Model file for the job. Use its own axes, mm. Face numbers are marked on the shaded views. A direction names the side the tool comes from. Give positions to 0.01 mm unless a question says otherwise; leave off trailing zeros. Write each loop counter-clockwise with the first axis right and the second up, starting at its lowest first coordinate (ties: lowest second). Pieces come first, ordered by that corner, then holes. Notation, with made-up numbers: (7, -17) - (13, -17) arc R21 ccw to (13, -9) - close; hole circle Ø1 at (4.5, -0.75). An arc over 180 degrees is marked (long way). Use CSV: the item, a comma, the result in double quotes.
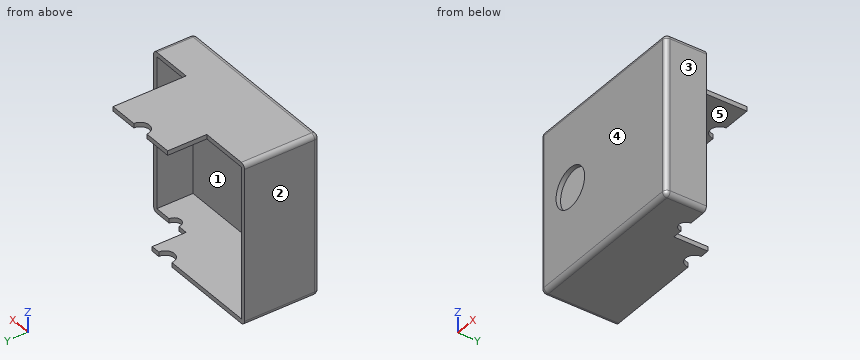
from build123d import *

# Parameters (mm, degrees)
SKETCH1_W           = 96
SKETCH1_H           = 89
BOSS_EXTRUDE1_DEPTH = 72.5
SKETCH3_W           = 91
SKETCH3_H           = 84
CUT_EXTRUDE1_DEPTH  = 70
SKETCH4_R           = 11
CUT_EXTRUDE3_DEPTH  = 10
CUT_EXTRUDE4_DEPTH  = 90
CUT_EXTRUDE5_DEPTH  = 10
SKETCH8_W           = 42
SKETCH8_H           = 21.66
BOSS_EXTRUDE2_DEPTH = 2.5
CUT_EXTRUDE6_DEPTH  = 2.5
FILLET1_R           = 2.5


with BuildPart() as part:
    # Sketch1 → Boss-Extrude1 (new body)
    with BuildSketch(Plane(origin=(0, 0, 0), x_dir=(1, 0, 0), z_dir=(0, 1, 0))):
        with Locations((48, -44.5)):
            Rectangle(SKETCH1_W, SKETCH1_H)
    extrude(amount=BOSS_EXTRUDE1_DEPTH)

    # Sketch3 → Cut-Extrude1 (cut)
    with BuildSketch(Plane(origin=(0, 72.5, 0), x_dir=(1, 0, 0), z_dir=(0, 1, 0))):
        with Locations((48, -44.5)):
            Rectangle(SKETCH3_W, SKETCH3_H)
    extrude(amount=-CUT_EXTRUDE1_DEPTH, mode=Mode.SUBTRACT)

    # Sketch4 → Cut-Extrude3 (cut)
    with BuildSketch(Plane.XZ):
        with Locations((22.7, 46)):
            Circle(SKETCH4_R)
    extrude(amount=-CUT_EXTRUDE3_DEPTH, mode=Mode.SUBTRACT)

    # Sketch6 → Cut-Extrude4 (cut, through all)
    with BuildSketch(Plane(origin=(0, 0, 0), x_dir=(-1, 0, 0), z_dir=(0, 0, -1))):
        Polygon((-96, 22.55), (-71, 22.55), (-71, 41.34), (0, 41.34), (0, 72.5), (-96, 72.5), align=None)
    extrude(amount=-CUT_EXTRUDE4_DEPTH, mode=Mode.SUBTRACT)

    # Sketch7 → Cut-Extrude5 (cut)
    with BuildSketch(Plane(origin=(0, 0, 0), x_dir=(-1, 0, 0), z_dir=(0, 0, -1))):
        with BuildLine():
            Line((-84, 22.55), (-76.5, 22.55))
            ThreePointArc((-76.5, 22.55), (-80.25, 18.8), (-84, 22.55))
        make_face()
        with BuildLine():
            Line((-65.9, 41.34), (-55.9, 41.34))
            ThreePointArc((-55.9, 41.34), (-60.9, 36.34), (-65.9, 41.34))
        make_face()
    extrude(amount=-CUT_EXTRUDE5_DEPTH, mode=Mode.SUBTRACT)

    # Sketch8 → Boss-Extrude2 (add)
    with BuildSketch(Plane.XY.offset(89)):
        with Locations((50, 52.17)):
            Rectangle(SKETCH8_W, SKETCH8_H)
    extrude(amount=-BOSS_EXTRUDE2_DEPTH)

    # Sketch9 → Cut-Extrude6 (cut)
    with BuildSketch(Plane.XY.offset(89)):
        with BuildLine():
            Line((45, 63), (55, 63))
            ThreePointArc((55, 63), (50, 58), (45, 63))
        make_face()
    extrude(amount=-CUT_EXTRUDE6_DEPTH, mode=Mode.SUBTRACT)

    # Fillet1
    fillet1_edges = [part.edges().sort_by_distance(p)[0] for p in [
        (0, 20.67, 0),
        (96, 11.275, 0),
        (96, 11.275, 89),
        (0, 20.67, 89),
        (48, 0, 0),
        (96, 0, 44.5),
        (48, 0, 89),
        (0, 0, 44.5),
    ]]
    fillet(fillet1_edges, radius=FILLET1_R)


solid = part.part
(1) Saw through at A-A, the plane x = 22.7. List the corners of the cut face in (y, z), then the cut area to 3 significant figures.
Checked values:
outline,"(0, 2.5) arc R2.5 ccw to (2.5, 0) - (41.34, 0) - (41.34, 2.5) - (2.5, 2.5) - (2.5, 35) - (0, 35) - close; (0, 57) - (2.5, 57) - (2.5, 86.5) - (41.34, 86.5) - (41.34, 89) - (2.5, 89) arc R2.5 ccw to (0, 86.5) - close"
area,"359 mm^2"
(2) Saw through at D-D, the plane z = 60.5. List the corners of the cut face in (x, y).
Checked values:
outline,"(0, 2.5) arc R2.5 ccw to (2.5, 0) - (93.5, 0) arc R2.5 ccw to (96, 2.5) - (96, 22.55) - (93.5, 22.55) - (93.5, 2.5) - (2.5, 2.5) - (2.5, 41.34) - (0, 41.34) - close"
(3) Flat gauge pins, fed straight in: P1, Ø2, axis at x = 69.5, z = 0.5, coming from the +Y side; P2, Ø0.8, axis at y = 42.5, z = 88, coming from the +X side; P3, Ø2, axis at x = 38, z = 38.5, coming from the +Y side. Where does each tip first touch, or does it go through?
Checked values:
P1,"stops at y = 41.34"
P2,"stops at x = 71"
P3,"stops at y = 2.5"
(4) Saw through at C-C, the plane x = 8.5. List the corners of the cut face in (y, z), then the cut area to 3 significant figures.
Checked values:
outline,"(0, 2.5) arc R2.5 ccw to (2.5, 0) - (41.34, 0) - (41.34, 2.5) - (2.5, 2.5) - (2.5, 86.5) - (41.34, 86.5) - (41.34, 89) - (2.5, 89) arc R2.5 ccw to (0, 86.5) - close"
area,"414 mm^2"
(5) Pull direction X, two halves, no side cores. Call the marked faces 1, 2 and 3: released by +X, released by -X, zero draft, split by the parting line, or undercut.
Checked values:
face 1,"undercut"
face 2,"released by -X"
face 3,"released by +X"
(6) Saw through at B-B, the plane y = 13. List the corners of the cut face in (x, z).
Checked values:
outline,"(0, 2.5) arc R2.5 ccw to (2.5, 0) - (93.5, 0) arc R2.5 ccw to (96, 2.5) - (96, 86.5) arc R2.5 ccw to (93.5, 89) - (2.5, 89) arc R2.5 ccw to (0, 86.5) - close; hole (2.5, 2.5) - (93.5, 2.5) - (93.5, 86.5) - (2.5, 86.5) - close"
(7) Wall check: probe 1 along X at (y, z) = (6, 75.5); probe 2 along Z at (x, y) = (58.5, 19); probe 3 along Y at (x, z) = (88, 51.5). Give the ranges that are in metal, low to high. Write a range as [from, to].
Checked values:
probe 1,"x = [0, 2.5], [93.5, 96]"
probe 2,"z = [0, 2.5], [86.5, 89]"
probe 3,"y = [0, 2.5]"
(8) 3-axis set-ups, long thin cutter, end or side, ignore diameter. For the marked faces 4 and 5: which of +Z, -Z, +X, -X, +Y, -Y reach the whole face in a straight line?
Checked values:
face 4,"+Z, -Z, +X, -X, -Y"
face 5,"+Y"
